Answer from the drawing. Dimensions are ordinates in mm from the lowest x, y and z of the part. A direction names the side the tool comes from. Round coordinates to 2 decimals unless told otherwise and drop trailing zeros. Loops run counter-clockwise (first coordinate to the right, second up) from the corner with the lowest first, then second, coordinate; pieces in that order, holes last. Notation, with made-up numbers: M -13,76.5 L 12,76.5 A24 ccw 12,94.5 Z; hole C -17.5,-38 d8. An arc over 180 degrees is marked long. Answer as CSV lines item,"result".
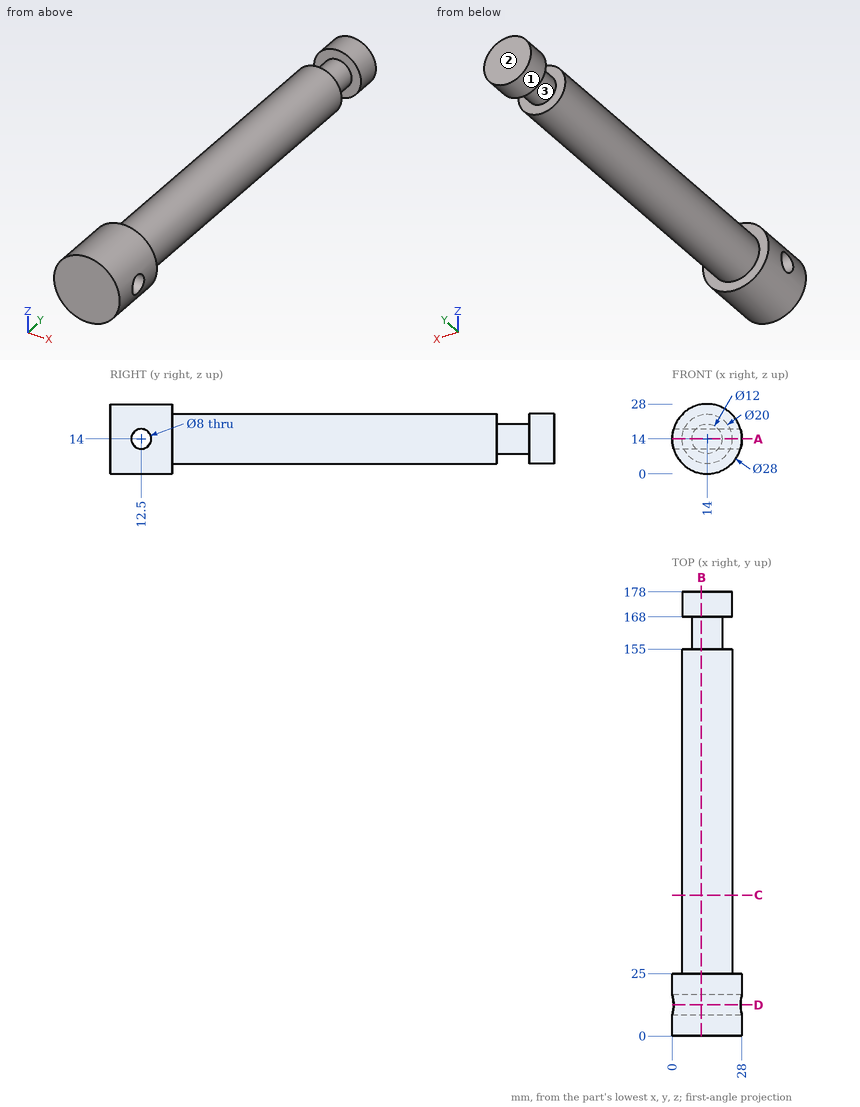
1) Find section A-A, the plane z = 14. Give the vertices of the cut face in (x, y).
Evaluation:
outline,"M 0,0 L 28,0 L 28,8.5 L 0,8.5 Z; M 0,16.5 L 28,16.5 L 28,25 L 24,25 L 24,155 L 20,155 L 20,168 L 24,168 L 24,178 L 4,178 L 4,168 L 8,168 L 8,155 L 4,155 L 4,25 L 0,25 Z"
2) Each of these flat-tipped pins is pushed along its axis until it touches: P1, Ø10, axis at y = 62.5, z = 13, coming from the -X side; P2, Ø4, axis at x = 13.5, y = 61, coming from the +Z side; P3, Ø3, axis at x = 19, y = 35.5, coming from the -Z side. Where does it stop, or does it pass through?
Evaluation:
P1,"stops at x = 4"
P2,"stops at z = 24"
P3,"stops at z = 4.63"
3) A tool of negligible diameter and unlimited length cuts with its end or side. For the marked faces 1, 2 and 3, from which of +Z, -Z, +X, -X, +Y, -Y can it reach the whole face along a straight path? Write none if from no direction.
Evaluation:
face 1,"+Y"
face 2,"+Z, -Z, +X, -X, +Y"
face 3,"none"
4) Find section C-C, the plane y = 56.5. Give the vertices of the cut face in (x, z).
Evaluation:
outline,"C 14,14 d20"
5) Find section D-D, the plane y = 12.5. Give the vertices of the cut face in (x, z).
Evaluation:
outline,"M 0.58,10 A14 ccw 27.42,10 Z; M 0.58,18 L 27.42,18 A14 ccw Z"
6) Find section B-B, the plane x = 11.75. Give the vertices of the cut face in (y, z).
Evaluation:
outline,"M 0,0.18 L 25,0.18 L 25,4.26 L 155,4.26 L 155,8.44 L 168,8.44 L 168,4.26 L 178,4.26 L 178,23.74 L 168,23.74 L 168,19.56 L 155,19.56 L 155,23.74 L 25,23.74 L 25,27.82 L 0,27.82 Z; hole C 12.5,14 d8"
7) Straight lines are drawn through the part: line 1 (Y direction, x = 13.5, z = 4.75); line 2 (Y direction, x = 14.5, z = 14.25); line 3 (Y direction, x = 4.5, z = 11.5). For each, find the intervals that lie inside material, in ascending order.
Evaluation:
line 1,"y = 0 to 155, 168 to 178"
line 2,"y = 0 to 8.51, 16.49 to 178"
line 3,"y = 0 to 9.38, 15.62 to 155, 168 to 178"
